Input: dimensioned drawing with shaded views. Units: mm. Origin: part minimum x, y, z. A direction names the side the tool comes from. Round coordinates to 2 decimals unless told otherwise and drop trailing zeros. Loops run counter-clockwise (first coordinate to the right, second up) from the corner with the lowest first, then second, coordinate; pieces in that order, holes last.
Item 1: Section query B-B on z = 18.5. Return loops of the section in (x, y).
Item 2: Section query D-D on x = 22. Return loops of the section in (y, z), then the cut area to 3 significant figures.
Item 3: Pull-direction query (X, two-part tool) for the marked faces 4, 5, 6 and 7; classes: released by +X, released by -X, zero draft, split by the parting line, or undercut.
Item 4: Section query C-C on x = 10.5. Return loops of the section in (y, z).
Item 5: Section query A-A on y = 51. Return loops of the section in (x, z).
Item 6: Ray query, L1, parallel to X at y = 15.5, z = 114; L2, parallel to X at y = 61.5, z = 93; L3, parallel to Y at x = 24.5, z = 43. Return the intervals inside material, ascending.
Item 7: Access query for the marked faces 1, 2 and 3. Directions: +Z, -Z, +X, -X, +Y, -Y. A direction counts if a zero-diameter tool reaches every point of the face in a straight line with its end or side. Return the directions, or none.
Item 8: First-contact query: P1, Ø3, axis at y = 41, z = 13, coming from the -X side; P2, Ø16.5, axis at x = 4, z = 45, coming from the +Y side; P3, Ø2, axis at y = 27, z = 26.5, coming from the +X side. Flat tips, straight axial feed; report the tip coordinate or a pass-through.
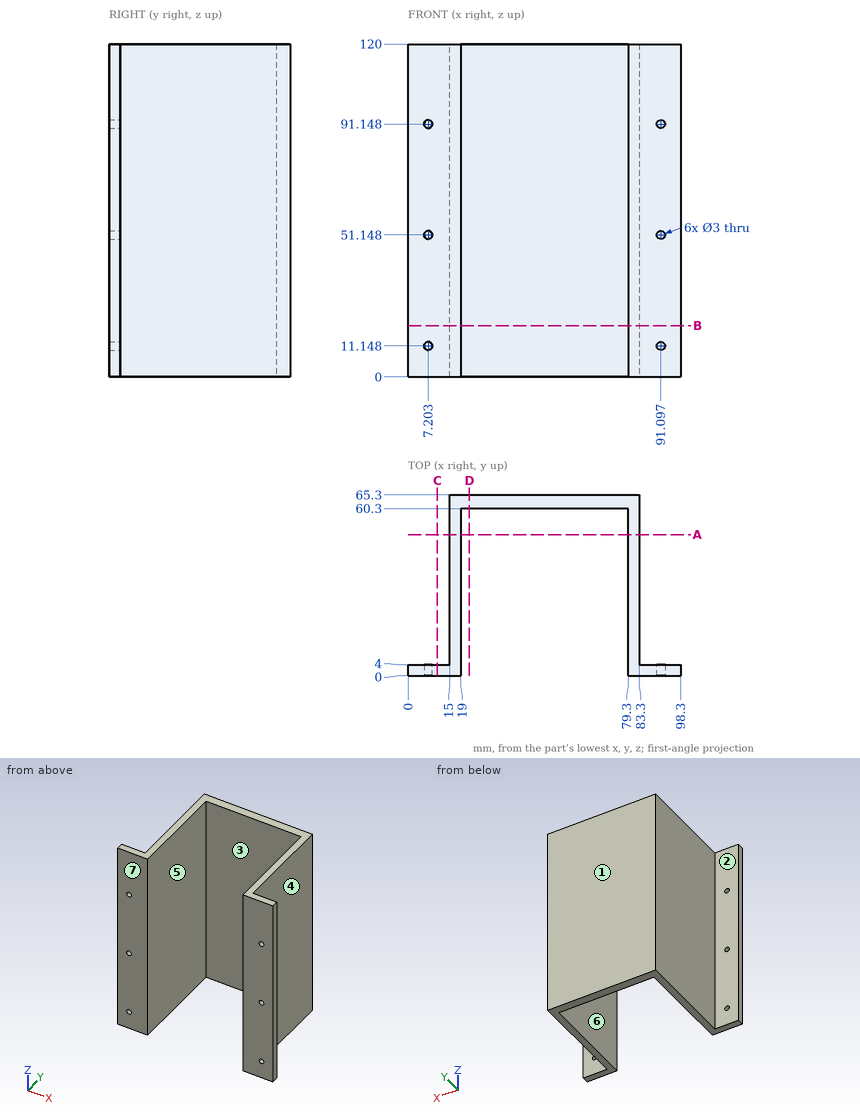
Data:
1. outline: (0, 0) - (19, 0) - (19, 60.3) - (79.3, 60.3) - (79.3, 0) - (98.3, 0) - (98.3, 4) - (83.3, 4) - (83.3, 65.3) - (15, 65.3) - (15, 4) - (0, 4) - close
2. outline: (60.3, 0) - (65.3, 0) - (65.3, 120) - (60.3, 120) - close
2. area: 600 mm2
3. face 4: released by +X
3. face 5: undercut
3. face 6: undercut
3. face 7: zero draft
4. outline: (0, 0) - (4, 0) - (4, 120) - (0, 120) - close
5. outline: (15, 0) - (19, 0) - (19, 120) - (15, 120) - close; (79.3, 0) - (83.3, 0) - (83.3, 120) - (79.3, 120) - close
6. L1: x = 15 to 19, 79.3 to 83.3
6. L2: x = 15 to 83.3
6. L3: y = 60.3 to 65.3
7. face 1: +Z, -Z, +X, -X, +Y
7. face 2: +Z, -Z, -X, +Y
7. face 3: +Z, -Z, -Y
8. P1: stops at x = 15
8. P2: stops at y = 4
8. P3: stops at x = 83.3
